Can you work these out from the model? Positions are in its coordinate system, mm. A direction names the side the tool comes from. Coordinates: 2 decimals unless noted, no trailing zeros. Order: outer loops, then holes, each group sorted by start corner. A loop starts at its lowest first (then second) coordinate and runs counter-clockwise, first axis right, second up. Notation, with made-up numbers: (35, 13.5) -> (66, 13.5) arc R19 cw to (66, 35.5) -> close; hole circle Ø11 at (28, 86). An arc over 180 degrees is marked (long way). Answer as a JSON object with one key per item and string values. Group by question number.
(1) I need wall thicknesses on line 1 (X direction, y = -0.25, z = 0); line 2 (Z direction, x = 3.25, y = -0.75); line 3 (Y direction, x = 2.75, z = 24.5). Which ranges of each line are inside material? Lowest first, please.
(2) If we mould it in two halves opening along Y, with no side actions, what happens to faces 1 (the cylindrical face through (-0.906, -2.877, 29.789)), 2 (the flat face through (0, 0, 32.147))? For each: pulls with the +Y half, pulls with the -Y half, needs draft (parallel to the pull), parting line crosses it, or undercut.
(3) I want a section at A-A, the plane z = 16.5. List the corners of the cut face in (x, y) for me (3 decimals), plus the area to 3 significant figures.
(4) For pin 1 (1.6 mm diameter, centred on x = -0.5, y = 0, fed in from +Z); pin 2 (2 mm diameter, centred on x = 3.5, z = 3, fed in from -Y), each with a flat end and sliding along its axis, tell me the tip position at first contact or that it passes through.
(5) Which directions (+Z, -Z, +X, -X, +Y, -Y) give clear straight access to the entire face, cutting with the end or side of a thin tool? Please do faces 3 (the cylindrical face through (2.8, -1.5, 1.7)), 4 (the cylindrical face through (1.03, -1.34, -27.62)), 5 (the cylindrical face through (4.65, 1.03, 33.13)), 6 (the flat face through (0.783, -1.381, 33.958)).
from build123d import *

# Parameters (mm, degrees)
CUT_EXTRUDE1_DEPTH = 3.571875


with BuildPart() as part:
    # Sketch4 → Revolve1 (revolve)
    with BuildSketch(Plane(origin=(0, 0, 0), x_dir=(0, 0, -1), z_dir=(1, 0, 0)), mode=Mode.PRIVATE) as revolve1_sk:
        Polygon((-30.95625, 4.7625), (-35.2425, 4.7625), (-35.71875, 4.28625), (-35.71875, 0), (26.19375, 0), (26.19375, 2.921), (25.93975, 3.175), (-28.59405, 3.175), (-28.7528, 3.01625), (-30.7975, 3.01625), (-30.95625, 3.175), align=None)
    revolve(revolve1_sk.sketch.rotate(Axis((0, 0, 35.71875), (0, 0, -1)), 180), axis=Axis((0, 0, 35.71875), (0, 0, -1)))

    # Sketch5 → Cut-Extrude1 (cut)
    with BuildSketch(Plane.XY.offset(35.71875)):
        Polygon((1.5875, 0.916543552), (0, 1.833087105), (-1.5875, 0.916543552), (-1.5875, -0.916543552), (0, -1.833087105), (1.5875, -0.916543552), align=None)
    extrude(amount=-CUT_EXTRUDE1_DEPTH, mode=Mode.SUBTRACT)

    # Cut-Extrude4 cone 1 section (on through the dimple's axis) → Cut-Extrude4 (revolve, cut)
    with BuildSketch(Plane(origin=(0, 0, 35.71875), x_dir=(0, -1, 0), z_dir=(1, 0, 0))):
        Polygon((0, 0), (1.833087105, 0), (0, 1.833087105), align=None)
    revolve(axis=Axis((0, 0, 35.71875), (0, 0, -1)), mode=Mode.SUBTRACT)

    # Sketch7 → Revolve2 (revolve)
    with BuildSketch(Plane(origin=(0, 0, 0), x_dir=(0, 0, -1), z_dir=(1, 0, 0))):
        Polygon((26.19375, 2.413), (34.925, 2.413), (35.71875, 1.61925), (35.71875, 0), (26.19375, 0), align=None)
    revolve(axis=Axis((0, 0, -35.71875), (0, 0, 1)))

    # Sketch10 → Cut-Revolve1 (revolve, cut)
    with BuildSketch(Plane(origin=(0, 0, 0), x_dir=(0, 0, -1), z_dir=(1, 0, 0))):
        with BuildLine():
            Line((26.91765, 1.6891), (28.30195, 1.6891))
            Line((28.30195, 1.6891), (29.78785, 3.175))
            Line((29.78785, 3.175), (26.19375, 3.175))
            Line((26.19375, 3.175), (26.19375, 2.413))
            ThreePointArc((26.19375, 2.413), (26.405775401, 1.901125401), (26.91765, 1.6891))
        make_face()
    revolve(axis=Axis((0, 0, -35.71875), (0, 0, 1)), mode=Mode.SUBTRACT)


solid = part.part
Computed values:
{
 "1": {"line 1": "x = -3.17 to 3.17", "line 2": "z = 30.96 to 35.72", "line 3": "y = -1.59 to 1.59"},
 "2": {"face 1": "parting line crosses it", "face 2": "undercut"},
 "3": {"outline": "circle Ø6.35 at (0, 0)", "area": "31.7 mm2"},
 "4": {"pin 1": "stops at z = 32.15", "pin 2": "stops at y = -1.96"},
 "5": {"face 3": "-Z", "face 4": "none", "face 5": "+Z, -Z", "face 6": "+Z"}
}
